```python
from build123d import *

# Parameters (mm, degrees)
SKETCH1_R           = 1.75
SKETCH1_R_2         = 3.5
BOSS_EXTRUDE3_DEPTH = 2
SKETCH3_R           = 1.5
CUT_EXTRUDE1_DEPTH  = 58.460820006


with BuildPart() as part:
    # Sketch1 → Boss-Extrude3 (new body)
    # profile 1 of 2: a face of its own
    with BuildSketch(Plane(origin=(0, 0, 0), x_dir=(1, 0, 0), z_dir=(0, 1, 0))):
        with BuildLine():
            ThreePointArc((40.05780493, 4.92208645), (19.51761867, 6.504088301), (-0.91087774, 3.843540262))
            ThreePointArc((-0.91087774, 3.843540262), (-3.626704772, -1.56509185), (2.171657179, -3.299455273))
            ThreePointArc((2.171657179, -3.299455273), (19.326940327, 1.634092765), (36.247955143, -4.051229892))
            ThreePointArc((36.247955143, -4.051229892), (38.163769521, -4.895969245), (40.257507506, -4.882165276))
            ThreePointArc((40.257507506, -4.882165276), (45.933967375, -5.003120525), (50.919436714, -7.720089844))
            ThreePointArc((50.919436714, -7.720089844), (50.66068815, -2.80185284), (55.57610439, -2.494136696))
            ThreePointArc((55.57610439, -2.494136696), (48.324550131, 2.276108307), (40.05780493, 4.92208645))
        make_face()
        with Locations(Location((0, 0, 0), (0, 0, 270))):
            Circle(SKETCH1_R, mode=Mode.SUBTRACT)
        with Locations(Location((39.178405, 0, 0), (0, 0, 270))):
            Circle(SKETCH1_R, mode=Mode.SUBTRACT)
    # profile 2 of 2: a face of its own
    with BuildSketch(Plane(origin=(0, 0, 0), x_dir=(1, 0, 0), z_dir=(0, 1, 0))):
        with Locations((53.273794312, -5.13030215)):
            Circle(SKETCH1_R_2)
    extrude(amount=BOSS_EXTRUDE3_DEPTH)

    # Sketch3 → Cut-Extrude1 (cut, through all)
    with BuildSketch(Plane(origin=(0, 2, 0), x_dir=(1, 0, 0), z_dir=(0, 1, 0))):
        with Locations(Location((53.273794312, -5.13030215, 0), (0, 0, 270))):
            Circle(SKETCH3_R)
    extrude(amount=-CUT_EXTRUDE1_DEPTH, mode=Mode.SUBTRACT)


solid = part.part
```
Work out the finished part from the listing and answer in its coordinate system (mm). Give positions to 0.01 mm unless a question says otherwise; leave off trailing zeros. Order: outer loops, then holes, each group sorted by start corner. A loop starts at its lowest first (then second) coordinate and runs counter-clockwise, first axis right, second up. Notation, with made-up numbers: M 14.5,19 L 49.5,19 A20 ccw 49.5,26 Z; hole C 21,85 d8. An arc over 180 degrees is marked long. Return JSON: item names as keys, results as strings.
1) This flat-tipped pin is pushed along its axis until it touches: pin 1 (1 mm diameter, centred on y = 0.5, z = 3, fed in from -X). Where does it stop, or does it pass through?
Resolved:
{"pin 1": "x = -3.06"}
2) Straight lines are drawn through the part: line 1 along X through (y, z) = (1.2, 1.5); line 2 along X through (y, z) = (0.5, 4.5); line 3 along X through (y, z) = (1.9, 1). For each, find the intervals that lie inside material, in ascending order. Write a range as [from, to].
Resolved:
{"line 1": "[-3.65, -0.9], [0.9, 5.3], [32.03, 38.28], [40.08, 54.38]", "line 2": "[37, 51.91], [54.63, 56.72]", "line 3": "[-3.82, -1.44], [1.44, 6.36], [30.97, 37.74], [40.61, 53.73]"}
3) For a pull along X with two mould halves and no side action, classify faces 1 (the cylindrical face through (55.83, 0.99, 7.52)), 2 (the flat face through (26, 0, -1)), 3 (the cylindrical face through (40.914, 0.986, -0.228)) as +X half, -X half, draft (parallel to the pull), parting line (faces both ways), or undercut.
Resolved:
{"face 1": "parting line", "face 2": "draft", "face 3": "undercut"}
4) Section B-B, the plane x = 0 is taken. Write down the section's boundary in (y, z).
Resolved:
{"outline": "M 0,-4.05 L 2,-4.05 L 2,-1.75 L 0,-1.75 Z; M 0,1.75 L 2,1.75 L 2,3.95 L 0,3.95 Z"}
5) Section A-A, the plane z = 0 is taken. Write down the section's boundary in (x, y), plus the area to 3 significant figures.
Resolved:
{"outline": "M -3.95,0 L -1.75,0 L -1.75,2 L -3.95,2 Z; M 1.75,0 L 8.88,0 L 8.88,2 L 1.75,2 Z; M 28.45,0 L 37.43,0 L 37.43,2 L 28.45,2 Z; M 40.93,0 L 52.32,0 L 52.32,2 L 40.93,2 Z", "area": "59.4 mm^2"}
6) Section D-D, the plane x = 35.5 is taken. Write down the section's boundary in (y, z).
Resolved:
{"outline": "M 0,-5.64 L 2,-5.64 L 2,3.53 L 0,3.53 Z"}
7) Section C-C, the plane y = 1.7 is taken. Write down the section's boundary in (x, z).
Resolved:
{"outline": "M -0.91,-3.84 A100 ccw 40.06,-4.92 A32 ccw 55.58,2.49 A3.5 ccw long 50.92,7.72 A12 cw 40.26,4.88 A5 ccw 36.25,4.05 A30 cw 2.17,3.3 A3.95 ccw long Z; hole C 0,0 d3.5; hole C 39.18,0 d3.5; hole C 53.27,5.13 d3"}
